Design review of the part shown in the three views and the two pictorial views. Dimensions are in mm from the part's minimum x, y and z. A direction names the side the tool comes from. Round coordinates to 2 decimals unless told otherwise and drop trailing zeros. Loops run counter-clockwise (first coordinate to the right, second up) from the corner with the lowest first, then second, coordinate; pieces in that order, holes last. Notation, with made-up numbers: M 22.25,-17.5 L 45.25,-17.5 A17 cw 45.25,-1.5 Z; hole C -4.5,72 d1. An arc over 180 degrees is marked long. One line per question, with ' | ' between items. Start each with the question number.
1) For probe 1 along X at (y, z) = (22.75, 60); probe 2 along Z at (x, y) = (25, 23.75), list the stretches that pass through material, from the lowest coordinate up. Write a range as from..to.
2) For pin 1 Ø7.5 at (y, z) = (16, 51) entering from -X, flat-tipped, find the tip position at first contact; note if it passes through.
3) We need section B-B (z = 69.5). Give the boundary of the cut face in (x, y).
4) For the marked faces 4 and 5, list the 3-axis set-ups (+Z, -Z, +X, -X, +Y, -Y) from which the entire face can be reached by the end or side of a thin tool; tool diameter is ignored.
5) We need section A-A (x = 20). Give the boundary of the cut face in (y, z).
6) Mouldability with a two-part tool opening along X and no side actions: class the marked faces 1, 2 and 3 as pulls with the +X half, pulls with the -X half, needs draft (parallel to the pull), parting line crosses it, or undercut.
7) We need section C-C (y = 19.25). Give the boundary of the cut face in (x, z), and give its area (3 significant figures).
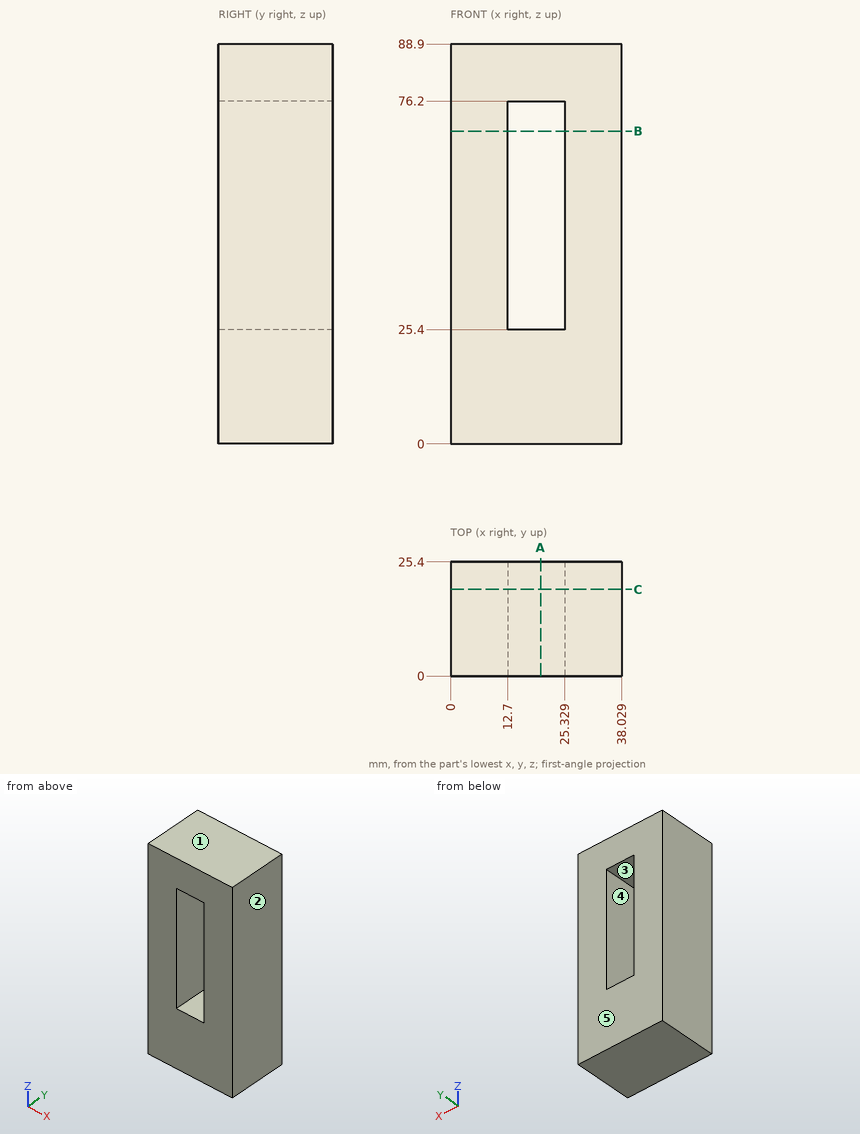
Answers below:
1) probe 1: 0..12.7, 25.33..38.03 | probe 2: 0..25.4, 76.2..88.9
2) pin 1: x = 0
3) outline: M 0,0 L 12.7,0 L 12.7,25.4 L 0,25.4 Z; M 25.33,0 L 38.03,0 L 38.03,25.4 L 25.33,25.4 Z
4) face 4: +Y, -Y | face 5: +Z, -Z, +X, -X, +Y
5) outline: M 0,0 L 25.4,0 L 25.4,25.4 L 0,25.4 Z; M 0,76.2 L 25.4,76.2 L 25.4,88.9 L 0,88.9 Z
6) face 1: needs draft | face 2: pulls with the +X half | face 3: undercut
7) outline: M 0,0 L 38.03,0 L 38.03,88.9 L 0,88.9 Z; hole M 12.7,25.4 L 25.33,25.4 L 25.33,76.2 L 12.7,76.2 Z | area: 2,740 mm^2
